```python
from build123d import *

# Parameters (mm, degrees)
F0_R     = 8
F1_DEPTH = 5
F3_DEPTH = 15
F5_DEPTH = 15
F7_DEPTH = 15


with BuildPart() as f1:
    # F0 (on Top) → F1 (new body)
    with BuildSketch(Plane.XY):
        with BuildLine():
            Line((2.5, 17.2409396496), (2.5, 19))
            Line((2.5, 19), (-2.5, 19))
            Line((-2.5, 19), (-2.5, 17.2409396496))
            Line((-2.5, 17.2409396496), (-4.3183749452, 9.0387803215))
            ThreePointArc((-4.3183749452, 9.0387803215), (-8.6753059831, 5.0086902446), (-9.9870008502, -0.7795677551))
            Line((-9.9870008502, -0.7795677551), (-16.1810917216, -6.4554063153))
            Line((-16.1810917216, -6.4554063153), (-17.7044826719, -7.3349364905))
            Line((-17.7044826719, -7.3349364905), (-15.2044826719, -11.6650635095))
            Line((-15.2044826719, -11.6650635095), (-13.6810917216, -10.7855333342))
            Line((-13.6810917216, -10.7855333342), (-5.668625905, -8.2592125663))
            ThreePointArc((-5.668625905, -8.2592125663), (0, -10.0173804893), (5.668625905, -8.2592125663))
            Line((5.668625905, -8.2592125663), (13.6810917216, -10.7855333342))
            Line((13.6810917216, -10.7855333342), (15.2044826719, -11.6650635095))
            Line((15.2044826719, -11.6650635095), (17.7044826719, -7.3349364905))
            Line((17.7044826719, -7.3349364905), (16.1810917216, -6.4554063153))
            Line((16.1810917216, -6.4554063153), (9.9870008502, -0.7795677551))
            ThreePointArc((9.9870008502, -0.7795677551), (8.6753059831, 5.0086902446), (4.3183749452, 9.0387803215))
            Line((4.3183749452, 9.0387803215), (2.5, 17.2409396496))
        make_face()
        Circle(F0_R, mode=Mode.SUBTRACT)
    extrude(amount=F1_DEPTH)

    # F2 (on face) → F3 (cut)
    with BuildSketch(Plane(origin=(16.4544826719, -9.5, 0), x_dir=(0.5, 0.8660254038, 0), z_dir=(0.8660254038, -0.5, 0))):
        with BuildLine():
            ThreePointArc((1.6, 2.5), (1.478207252, 3.1122934918), (1.1313708499, 3.6313708499))
            Line((1.1313708499, 3.6313708499), (-1.1313708499, 1.3686291501))
            ThreePointArc((-1.1313708499, 1.3686291501), (0.6122934918, 1.021792748), (1.6, 2.5))
        make_face()
        with BuildLine():
            Line((-1.1313708499, 1.3686291501), (1.1313708499, 3.6313708499))
            ThreePointArc((1.1313708499, 3.6313708499), (-1.1313708499, 3.6313708499), (-1.1313708499, 1.3686291501))
        make_face()
    extrude(amount=-F3_DEPTH, mode=Mode.SUBTRACT)

    # F4 (on face) → F5 (cut)
    with BuildSketch(Plane(origin=(0, 19, 0), x_dir=(-1, 0, 0), z_dir=(0, 1, 0))):
        with BuildLine():
            Line((-1.1313708499, 3.6313708499), (1.1313708499, 1.3686291501))
            ThreePointArc((1.1313708499, 1.3686291501), (1.478207252, 1.8877065082), (1.6, 2.5))
            ThreePointArc((1.6, 2.5), (0.6122934918, 3.978207252), (-1.1313708499, 3.6313708499))
        make_face()
        with BuildLine():
            ThreePointArc((-1.1313708499, 3.6313708499), (-1.1313708499, 1.3686291501), (1.1313708499, 1.3686291501))
            Line((1.1313708499, 1.3686291501), (-1.1313708499, 3.6313708499))
        make_face()
    extrude(amount=-F5_DEPTH, mode=Mode.SUBTRACT)

    # F6 (on face) → F7 (cut)
    with BuildSketch(Plane(origin=(-16.4544826719, -9.5, 0), x_dir=(0.5, -0.8660254038, 0), z_dir=(-0.8660254038, -0.5, 0))):
        with BuildLine():
            ThreePointArc((1.1313708499, 3.6313708499), (-1.1313708499, 3.6313708499), (-1.1313708499, 1.3686291501))
            Line((-1.1313708499, 1.3686291501), (1.1313708499, 3.6313708499))
        make_face()
        with BuildLine():
            Line((1.1313708499, 3.6313708499), (-1.1313708499, 1.3686291501))
            ThreePointArc((-1.1313708499, 1.3686291501), (0.6122934918, 1.021792748), (1.6, 2.5))
            ThreePointArc((1.6, 2.5), (1.478207252, 3.1122934918), (1.1313708499, 3.6313708499))
        make_face()
    extrude(amount=-F7_DEPTH, mode=Mode.SUBTRACT)


solid = f1.part
```
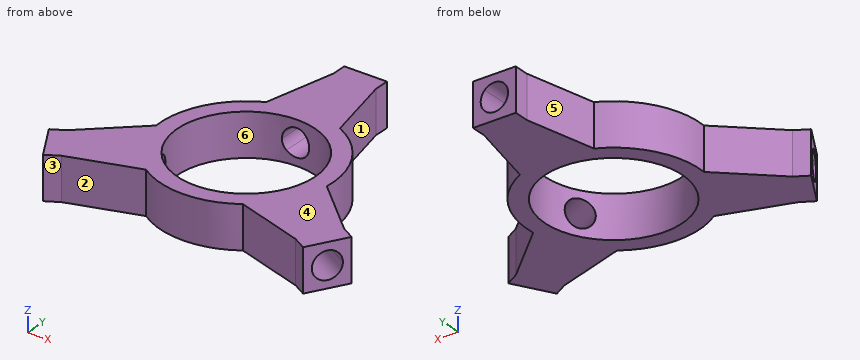
Check sheet for the modelled part. Datum: model origin and axes. Units: mm. Face numbers are marked on the shaded views. A direction names the side the tool comes from. Round coordinates to 2 decimals unless told otherwise and drop trailing zeros. Order: outer loops, then holes, each group sorted by start corner. A loop starts at its lowest first (then second) coordinate and runs counter-clockwise, first axis right, second up. Notation, with made-up numbers: (27, 68.25) - (42, 68.25) arc R4 ccw to (42, 75.25) - close; hole circle Ø8 at (66.5, 51). An arc over 180 degrees is marked (long way). Write item = value, one per line.
Q1. Section check C-C (z = 3.2). State how many separate pieces and enclosed holes the cut face has, and give its area (3 significant figures).
Computed:
separate_pieces = 3
enclosed_holes = 0
area = 196 mm^2
Q2. Thickness scan on line 1 along X through (y, z) = (17.5, 2.55); line 2 along Y through (x, z) = (0, 3.1); line 3 along Z through (x, y) = (-12, -7). Record the ranges inside material, lowest first.
Computed:
line_1 = -2.5 to -1.6, 1.6 to 2.5
line_2 = -10.02 to -8
line_3 = 0 to 0.9, 4.1 to 5
Q3. Go/stop test with flat-tipped pins: pin 1 (2 mm diameter, centred on x = 9.5, z = 1, fed in from +Y); pin 2 (2 mm diameter, centred on y = -4.5, z = 2, fed in from -X); pin 3 (3 mm diameter, centred on y = 11, z = 1, fed in from -X); pin 4 (8 mm diameter, centred on x = -6, y = -2, fed in from -Z). Record where each tip stops, or that it passes through.
Computed:
pin_1 = 5.3
pin_2 = -15.14
pin_3 = -4.22
pin_4 = 0
Q4. Section check B-B (y = 0). Record the boundary of the cut face in (x, z), and give its area (3 significant figures).
Computed:
outline = (-10.02, 0) - (-8, 0) - (-8, 5) - (-10.02, 5) - close; (8, 0) - (10.02, 0) - (10.02, 5) - (8, 5) - close
area = 20.2 mm^2
Q5. Section check A-A (x = 0). Record the boundary of the cut face in (y, z), and give its area (3 significant figures).
Computed:
outline = (-10.02, 0) - (-8, 0) - (-8, 5) - (-10.02, 5) - close; (8, 0) - (19, 0) - (19, 0.9) - (8, 0.9) - close; (8, 4.1) - (19, 4.1) - (19, 5) - (8, 5) - close
area = 29.9 mm^2
Q6. Tool access check on the marked faces 1 and 2. Record the directions out of +Z, -Z, +X, -X, +Y, -Y that give a thin tool (end or side, any length) a straight path to the whole face; none if there is none.
Computed:
face_1 = +Z, -Z, +X, +Y
face_2 = +Z, -Z, -Y
Q7. Draft check along Y on the marked faces 3, 4, 5 and 6. Enter one of: pulls with the +Y half, pulls with the -Y half, needs draft (parallel to the pull), parting line crosses it, or undercut.
Computed:
face_3 = pulls with the -Y half
face_4 = needs draft
face_5 = pulls with the +Y half
face_6 = undercut
Q8. Section check D-D (y = 10). Record the boundary of the cut face in (x, z), and give its area (3 significant figures).
Computed:
outline = (-4.11, 0) - (4.11, 0) - (4.11, 5) - (-4.11, 5) - close; hole circle Ø3.2 at (0, 2.5)
area = 33.0 mm^2
